Autodesk Inventor part; units mm, degrees
sketch "Sketch1" plane through (0, 0, 0) normal (0, 0, 1) x (1, 0, 0)
  line L0 (-100, 100) -> (100, 100)
  arc A0 (-100, 100) -> (-194.8683, 0) centre (-100, 5) ccw
  arc A1 (194.8683, 0) -> (100, 100) centre (100, 5) ccw
  arc A2 (-100, 95) -> (-189.861, 0) centre (-100, 5) ccw
  line L1 (-100, 95) -> (100, 95)
  arc A3 (189.861, 0) -> (100, 95) centre (100, 5) ccw
  line L2 (-194.8683, 0) -> (-189.861, 0)
  line L3 (189.861, 0) -> (194.8683, 0)
  point P0 (0, 0)
  point P1 (0, 100)
  dimension "d0" = 200
  dimension "d1" = 100
  dimension "d3" = 5
  dimension "d9" = 90
extrude "Extrusion1" add sketch "Sketch1" along normal mid plane 200
properties part number "Sessao_28_03_003_001" material "Wood (Walnut)"
Input: part model. Units: mm. Frame: model coordinates. A direction names the side the tool comes from. Round coordinates to 2 decimals unless told otherwise and drop trailing zeros. Loops run counter-clockwise (first coordinate to the right, second up) from the corner with the lowest first, then second, coordinate; pieces in that order, holes last.
1) Set-up query: faces 4 (the flat face through (-15, 98, 100)), 5 (the flat face through (-1, 95, -1)). Return all of +Z, -Z, +X, -X, +Y, -Y with unobstructed straight access to the full face (end or side cutting, diameter ignored); none if empty.
Ans:
face 4: +Z, +X, -X, +Y, -Y
face 5: +Z, -Z, -Y
2) Section query D-D on y = 41. Return the cut outline in (x, z).
Ans:
outline: (-187.91, -100) - (-182.49, -100) - (-182.49, 100) - (-187.91, 100) - close; (182.49, -100) - (187.91, -100) - (187.91, 100) - (182.49, 100) - close
3) Section query A-A on y = 64. Return the cut outline in (x, z).
Ans:
outline: (-174.46, -100) - (-167.96, -100) - (-167.96, 100) - (-174.46, 100) - close; (167.96, -100) - (174.46, -100) - (174.46, 100) - (167.96, 100) - close
4) Material intervals for line 1 (X direction, y = 11, z = -69); line 2 (X direction, y = 8.5, z = 61); line 3 (Y direction, x = -66.5, z = -20), sorted ascending.
Ans:
line 1: x = -194.81 to -189.8, 189.8 to 194.81
line 2: x = -194.94 to -189.93, 189.93 to 194.94
line 3: y = 95 to 100
5) Section query B-B on z = 72.5. Return the cut outline in (x, y), plus the area to 3 significant figures.
Ans:
outline: (-194.87, 0) - (-189.86, 0) arc R90 cw to (-100, 95) - (100, 95) arc R90 cw to (189.86, 0) - (194.87, 0) arc R95 ccw to (100, 100) - (-100, 100) arc R95 ccw to start
area: 2,500 mm2
6) Section query C-C on x = -74.5. Return the cut outline in (y, z), plus the area to 3 significant figures.
Ans:
outline: (95, -100) - (100, -100) - (100, 100) - (95, 100) - close
area: 1,000 mm2
7) Pin query (flat end, axial travel): pin 1 (2 mm diameter, centred on x = -66, z = -4, fed in from -Y); pin 2 (1.5 mm diameter, centred on x = 121.5, z = 66.5, fed in from +Y); pin 3 (12 mm diameter, centred on x = -105, z = -23.5, fed in from +Y). Return the tip coordinate at first contact, or that it passes through.
Ans:
pin 1: stops at y = 95
pin 2: stops at y = 97.71
pin 3: stops at y = 100
8) Pull-direction query (X, two-part tool) for faces 1 (the cylindrical face through (-169.659, 69.596, -1.4)), 2 (the flat face through (-1, 100, -1)), 3 (the cylindrical face through (164.675, 67.587, -1.4)); classes: released by +X, released by -X, zero draft, split by the parting line, or undercut.
Ans:
face 1: released by -X
face 2: zero draft
face 3: undercut
